Can you work these out from the model? Positions are in its coordinate system, mm. A direction names the side the tool comes from. Round coordinates to 2 decimals unless told otherwise and drop trailing zeros. Loops run counter-clockwise (first coordinate to the right, second up) from the corner with the lowest first, then second, coordinate; pieces in that order, holes last. Notation, with made-up numbers: M 20,-34 L 44,-34 A18 cw 44,-21 Z; hole C -32,84.5 d6. An arc over 180 degrees is marked long. Return JSON: item names as keys, results as strings.
```python
from build123d import *

# Parameters (mm, degrees)
BOSS_EXTRUDE1_DEPTH = 1.4
SKETCH2_OUTSIDE_W   = 18.618
SKETCH2_OUTSIDE_H   = 17.226
SKETCH2_OUTSIDE_R   = 4.5
CUT_EXTRUDE1_DEPTH  = 1
CUT_EXTRUDE1_TAPER  = 60
SKETCH3_R           = 2.425
BOSS_EXTRUDE2_DEPTH = 24.3
SKETCH4_OUTSIDE_W   = 18.218
SKETCH4_OUTSIDE_H   = 16.826
SKETCH4_OUTSIDE_R   = 1.95
CUT_EXTRUDE2_DEPTH  = 2.5
SKETCH5_R           = 2.6
BOSS_EXTRUDE3_DEPTH = 11.5


with BuildPart() as part:
    # Sketch1 → Boss-Extrude1 (new body)
    with BuildSketch(Plane(origin=(0, 0, 0), x_dir=(1, 0, 0), z_dir=(0, 1, 0))):
        Polygon((5.195, 0), (2.5975, 4.499001973), (-2.5975, 4.499001973), (-5.195, 0), (-2.5975, -4.499001973), (2.5975, -4.499001973), align=None)
    extrude(amount=BOSS_EXTRUDE1_DEPTH)

    # Sketch2 outside → Cut-Extrude1 (cut)
    with BuildSketch(Plane(origin=(0, 1.4, 0), x_dir=(1, 0, 0), z_dir=(0, 1, 0))):
        Rectangle(SKETCH2_OUTSIDE_W, SKETCH2_OUTSIDE_H)
        Circle(SKETCH2_OUTSIDE_R, mode=Mode.SUBTRACT)
    extrude(amount=-CUT_EXTRUDE1_DEPTH, taper=CUT_EXTRUDE1_TAPER, mode=Mode.SUBTRACT)

    # Sketch3 → Boss-Extrude2 (add)
    with BuildSketch(Plane.XZ):
        Circle(SKETCH3_R)
    extrude(amount=BOSS_EXTRUDE2_DEPTH)

    # Sketch4 outside → Cut-Extrude2 (cut)
    with BuildSketch(Plane.XZ.offset(24.3)):
        Rectangle(SKETCH4_OUTSIDE_W, SKETCH4_OUTSIDE_H)
        Circle(SKETCH4_OUTSIDE_R, mode=Mode.SUBTRACT)
    extrude(amount=-CUT_EXTRUDE2_DEPTH, mode=Mode.SUBTRACT)

    # Sketch5 → Boss-Extrude3 (add)
    with BuildSketch(Plane.XZ):
        Circle(SKETCH5_R)
    extrude(amount=BOSS_EXTRUDE3_DEPTH)


solid = part.part
```
Q1. Suppose I cut it at B-B, the plane y = -16.5. Please give me the cut outline in (x, z) (3 decimals), plus the area to 3 significant figures.
Results:
{"outline": "C 0,0 d4.85", "area": "18.5 mm2"}
Q2. If I drill on line 1 along Y through (x, z) = (-2.25, -2); line 2 along Z through (x, y) = (2.25, -1); line 3 along Z through (x, y) = (1.75, -1), over which ranges is the centre line in solid material (lowest first)?
Results:
{"line 1": "y = 0 to 1.4", "line 2": "z = -1.3 to 1.3", "line 3": "z = -1.92 to 1.92"}
Q3. Suppose I cut it at A-A, the plane y = -9.5. Please give me the cut outline in (x, z), plus the area to 3 significant figures.
Results:
{"outline": "C 0,0 d5.2", "area": "21.2 mm2"}
Q4. On a 3-axis mill with a long thin cutter (end or side, diameter ignored), from which of +Z, -Z, +X, -X, +Y, -Y can I reach the whole of each face in a straight line? I mean faces 1 (the cylindrical face through (-1.437, -23.068, 1.318)), 2 (the conical face through (2.325, 1.302, -4.049)). Say none if no direction works.
Results:
{"face 1": "-Y", "face 2": "-Z, +X, +Y"}
Q5. I'm going to push flat-ended pins straight in: pin 1 Ø5 at (y, z) = (-11.5, -1) entering from -X; pin 2 Ø1 at (y, z) = (-6, 0.5) entering from +X; pin 3 Ø5 at (x, z) = (-4, -0.5) entering from -Y; pin 4 Ø5 at (x, y) = (-3.5, -17.5) entering from +Z. Where does each tip first touch, or does it pass through?
Results:
{"pin 1": "stops at x = -2.6", "pin 2": "stops at x = 2.6", "pin 3": "stops at y = -24.3", "pin 4": "stops at z = 2.21"}
